For this review, take the finished solid that the model builds, in its own axes (mm). A direction names the side the tool comes from. Give positions to 0.01 mm unless a question says otherwise; leave off trailing zeros. Loops run counter-clockwise (first coordinate to the right, second up) from the corner with the lowest first, then second, coordinate; pieces in that order, holes last. Notation, with made-up numbers: M 68,1.25 L 123,1.25 A16 ccw 123,27.25 Z; hole C 84,34 d11. An arc over 180 degrees is marked long. Use CSV: the item, a comma, the result in double quotes. Start each with the question number.
1. Insertion check: P1, Ø3, axis at y = -5, z = -21.5, coming from the +X side; P2, Ø4.5, axis at x = 5.48, z = -5.65, coming from the +Y side; P3, Ø18.5, axis at x = 22, z = -19.5, coming from the +Y side; P4, Ø7.5, axis at x = 8, y = -2.5, coming from the -Z side. Each pin has a flat end and moves straight along its axis. Give the tip position at first contact, or say it passes through.
2. Tool access review of faces 1 (the face through (16, -12.7, -19)), 2 (the face through (14, 0, -23)), 3 (the face through (-3.69, -6, -12)): name each direction out of +Z, -Z, +X, -X, +Y, -Y from which nothing blocks a thin tool from reaching the whole face with its end or side.
3. Take a section at A-A, the plane x = 6.5. Write out the cut boundary in (y, z), and give its area (3 significant figures).
4. Take a section at B-B, the plane y = -10.5. Write out the cut boundary in (x, z) (3 decimals), and give its area (3 significant figures).
5. Take a section at C-C, the plane x = -5. Write out the cut boundary in (y, z).
6. Take a section at D-D, the plane z = -14. Write out the cut boundary in (x, y), and give its area (3 significant figures).
7. To check wall thickness, follow line 1 (Z direction, x = 5.5, y = 6.5); line 2 (Z direction, x = -3, y = 4.5); line 3 (Z direction, x = 24, y = 2.25). State the ranges of each line that lie inside material, in increasing order. Write a range as [from, to].
from build123d import *

# Parameters (mm, degrees)
F0_R     = 1.905
F1_DEPTH = 12.7
F2_DEPTH = 12.7
F3_DEPTH = 12.7


with BuildPart() as f1:
    # F0 (on Front) → F1 (new body)
    with BuildSketch(Plane.XZ):
        Polygon((-3.6898989651, -8.8297099552), (32.9718431285, -8.8297099552), (32.9718431285, -2.4797099552), (-3.6898989651, -2.4797099552), (-3.6898989651, -5.6547099552), align=None)
        with Locations((5.4755365583, -5.6547099552)):
            Circle(F0_R, mode=Mode.SUBTRACT)
        with Locations((23.8064076051, -5.6547099552)):
            Circle(F0_R, mode=Mode.SUBTRACT)
        Polygon((14.6409720817, -46.9297099552), (32.9718431285, -15.1797099552), (32.9718431285, -8.8297099552), (-3.6898989651, -8.8297099552), (-3.6898989651, -15.1797099552), align=None)
        with BuildLine():
            ThreePointArc((-6.8648989651, -8.8297099552), (-4.6198349348, -7.8997739855), (-3.6898989651, -5.6547099552))
            ThreePointArc((-3.6898989651, -5.6547099552), (-4.6198349348, -3.409645925), (-6.8648989651, -2.4797099552))
            ThreePointArc((-6.8648989651, -2.4797099552), (-10.0398989651, -5.6547099552), (-6.8648989651, -8.8297099552))
        make_face()
        with Locations((-6.8648989651, -5.6547099552)):
            Circle(F0_R, mode=Mode.SUBTRACT)
        with BuildLine():
            Line((-3.6898989651, -5.6547099552), (-3.6898989651, -2.4797099552))
            Line((-3.6898989651, -2.4797099552), (-6.8648989651, -2.4797099552))
            ThreePointArc((-6.8648989651, -2.4797099552), (-4.6198349348, -3.409645925), (-3.6898989651, -5.6547099552))
        make_face()
        with BuildLine():
            Line((-6.8648989651, -8.8297099552), (-3.6898989651, -8.8297099552))
            Line((-3.6898989651, -8.8297099552), (-3.6898989651, -5.6547099552))
            ThreePointArc((-3.6898989651, -5.6547099552), (-4.6198349348, -7.8997739855), (-6.8648989651, -8.8297099552))
        make_face()
        with Locations((-6.8648989651, -5.6547099552)):
            Circle(F0_R)
    extrude(amount=F1_DEPTH)

    # F0 (on Front) → F2 (join)
    with BuildSketch(Plane.XZ):
        Polygon((-3.6898989651, -8.8297099552), (32.9718431285, -8.8297099552), (32.9718431285, -2.4797099552), (-3.6898989651, -2.4797099552), (-3.6898989651, -5.6547099552), align=None)
        with Locations((5.4755365583, -5.6547099552)):
            Circle(F0_R, mode=Mode.SUBTRACT)
        with Locations((23.8064076051, -5.6547099552)):
            Circle(F0_R, mode=Mode.SUBTRACT)
        with BuildLine():
            ThreePointArc((-6.8648989651, -8.8297099552), (-4.6198349348, -7.8997739855), (-3.6898989651, -5.6547099552))
            ThreePointArc((-3.6898989651, -5.6547099552), (-4.6198349348, -3.409645925), (-6.8648989651, -2.4797099552))
            ThreePointArc((-6.8648989651, -2.4797099552), (-10.0398989651, -5.6547099552), (-6.8648989651, -8.8297099552))
        make_face()
        with Locations((-6.8648989651, -5.6547099552)):
            Circle(F0_R, mode=Mode.SUBTRACT)
        with BuildLine():
            Line((-3.6898989651, -5.6547099552), (-3.6898989651, -2.4797099552))
            Line((-3.6898989651, -2.4797099552), (-6.8648989651, -2.4797099552))
            ThreePointArc((-6.8648989651, -2.4797099552), (-4.6198349348, -3.409645925), (-3.6898989651, -5.6547099552))
        make_face()
        with BuildLine():
            Line((-6.8648989651, -8.8297099552), (-3.6898989651, -8.8297099552))
            Line((-3.6898989651, -8.8297099552), (-3.6898989651, -5.6547099552))
            ThreePointArc((-3.6898989651, -5.6547099552), (-4.6198349348, -7.8997739855), (-6.8648989651, -8.8297099552))
        make_face()
    extrude(amount=-F2_DEPTH)

    # F0 (on Front) → F3 (join)
    with BuildSketch(Plane.XZ):
        with Locations((-6.8648989651, -5.6547099552)):
            Circle(F0_R)
    extrude(amount=-F3_DEPTH)


solid = f1.part
Result set:
1,P1,"x = 30.19"
1,P2,"y = 12.7"
1,P3,"y = 0"
1,P4,"z = -41.92"
2,face 1,"+Z, -Z, +X, -X, -Y"
2,face 2,"-Z, +X, -X, +Y"
2,face 3,"-Z, -X, +Y, -Y"
3,outline,"M -12.7,-32.83 L 0,-32.83 L 0,-8.83 L 12.7,-8.83 L 12.7,-7.26 L -12.7,-7.26 Z; M -12.7,-4.05 L 12.7,-4.05 L 12.7,-2.48 L -12.7,-2.48 Z"
3,area,"384 mm2"
4,outline,"M -6.865,-8.83 L -3.69,-8.83 L -3.69,-15.18 L 14.641,-46.93 L 32.972,-15.18 L 32.972,-2.48 L -6.865,-2.48 A3.175 ccw Z; hole C 5.476,-5.655 d3.81; hole C 23.806,-5.655 d3.81"
4,area,"1,060 mm2"
5,outline,"M -12.7,-8.83 L 12.7,-8.83 L 12.7,-2.48 L -12.7,-2.48 Z"
6,outline,"M -3.69,-12.7 L 32.97,-12.7 L 32.97,0 L -3.69,0 Z"
6,area,"466 mm2"
7,line 1,"[-8.83, -7.56], [-3.75, -2.48]"
7,line 2,"[-8.83, -2.48]"
7,line 3,"[-8.83, -7.55], [-3.76, -2.48]"
